The listing builds one solid part. Answer for the finished solid, in the listing's coordinates (mm). Face numbers are marked on the shaded views. A direction names the side the tool comes from. Coordinates: 2 decimals unless noted, no trailing zeros. Write each loop counter-clockwise with the first axis right and the second up, starting at its lowest first coordinate (ties: lowest second). Pieces come first, ordered by that corner, then holes.
(1) The part is cut by section C-C on y = 7.25. Determine the outline of the cut face in (x, z), plus the area to 3 significant figures.
(2) The part is cut by section B-B on y = 3.75. Determine the outline of the cut face in (x, z).
(3) Which of the six approach directions +Z, -Z, +X, -X, +Y, -Y give full straight-line access (tool end or side, diameter ignored) to the marked faces 1 and 2?
(4) Straight lines are drawn through the part: line 1 (X direction, y = 8.75, z = 1.15); line 2 (Y direction, x = -2, z = -0.9); line 3 (X direction, y = 1.5, z = 0.65). For each, find the intervals that lie inside material, in ascending order.
(5) For a pull along X with two mould halves and no side action, classify the marked faces 3, 4 and 5 as +X half, -X half, draft (parallel to the pull), parting line (faces both ways), or undercut.
(6) Given P1, Ø4, axis at x = -3, y = 2.5, coming from the -Z side, flat-ended and moving along its own axis, determine where the tip first touches the part or whether it passes through.
(7) The part is cut by section D-D on x = 5.5. Determine the outline of the cut face in (y, z).
(8) The part is cut by section A-A on z = 0.4. Determine the outline of the cut face in (x, y), plus the area to 3 significant figures.
from build123d import *

# Parameters (mm, degrees)
F1_DEPTH = 2.54
F2_R     = 2.53999
F4_D     = 4.064
F4_DEPTH = 12.5231992362
F5_D     = 4.064


# Not quite as in the source:
# - a fillet or chamfer is up to 0.001 mm smaller than in the source, because OpenCascade refuses the exact size


with BuildPart() as f1:
    # F0 (on Top) → F1 (new body, symmetric)
    with BuildSketch(Plane.XY):
        with BuildLine():
            Line((-12.5221992362, 9.4272772469), (-12.5221992362, 8.3157558613))
            Line((-12.5221992362, 8.3157558613), (-12.5221992362, 2.3621992362))
            ThreePointArc((-12.5221992362, 2.3621992362), (-11.8303270984, 0.6918721378), (-10.16, 0))
            Line((-10.16, 0), (0, 0))
            Line((0, 0), (10.16, 0))
            ThreePointArc((10.16, 0), (11.8303270984, 0.6918721378), (12.5221992362, 2.3621992362))
            Line((12.5221992362, 2.3621992362), (12.5221992362, 8.3157558613))
            Line((12.5221992362, 8.3157558613), (12.5221992362, 9.4272772469))
            Line((12.5221992362, 9.4272772469), (11.43, 9.4272772469))
            Line((11.43, 9.4272772469), (11.43, 8.3157558613))
            Line((11.43, 8.3157558613), (11.43, 2.3621992362))
            ThreePointArc((11.43, 2.3621992362), (11.0580256121, 1.464173624), (10.16, 1.0921992362))
            Line((10.16, 1.0921992362), (1.2192031136, 1.0921992362))
            Line((1.2192031136, 1.0921992362), (0, 1.0921992362))
            Line((0, 1.0921992362), (-10.16, 1.0921992362))
            ThreePointArc((-10.16, 1.0921992362), (-11.0580256121, 1.464173624), (-11.43, 2.3621992362))
            Line((-11.43, 2.3621992362), (-11.43, 8.3157558613))
            Line((-11.43, 8.3157558613), (-11.43, 9.4272772469))
            Line((-11.43, 9.4272772469), (-12.5221992362, 9.4272772469))
        make_face()
    extrude(amount=F1_DEPTH, both=True)

    # F2 (radius 2.54 in the source; OpenCascade refuses exactly that, so slightly less here)
    f2_edges = [f1.edges().sort_by_distance(p)[0] for p in [
        (-11.9761, 9.427277, 2.54),
        (-11.9761, 9.427277, -2.54),
        (11.9761, 9.427277, 2.54),
        (11.9761, 9.427277, -2.54),
    ]]
    fillet(f2_edges, radius=F2_R)

    # F4 (through all, one way)
    with BuildSketch(Plane(origin=(0, 0, 0), x_dir=(0, 1, 0), z_dir=(-1, 0, 0))):
        with Locations((6.2061757781, 0)):
            Circle(F4_D / 2)
    extrude(amount=-F4_DEPTH, mode=Mode.SUBTRACT)

    # F5 (through all)
    with Locations(Plane.YZ):
        with Locations((6.2061757781, 0)):
            Hole(F5_D / 2)


solid = f1.part
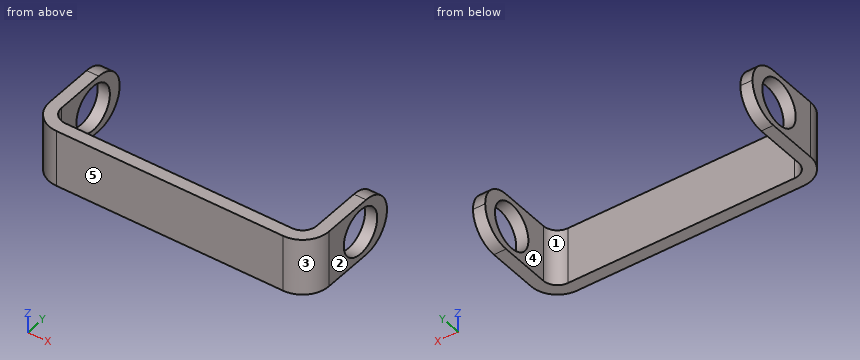
Model answer:
1. outline: (-12.52, -2.51) - (-11.43, -2.51) - (-11.43, -1.74) - (-12.52, -1.74) - close; (-12.52, 1.74) - (-11.43, 1.74) - (-11.43, 2.51) - (-12.52, 2.51) - close; (11.43, -2.51) - (12.52, -2.51) - (12.52, -1.74) - (11.43, -1.74) - close; (11.43, 1.74) - (12.52, 1.74) - (12.52, 2.51) - (11.43, 2.51) - close
1. area: 3.37 mm2
2. outline: (-12.52, -2.54) - (-11.43, -2.54) - (-11.43, 2.54) - (-12.52, 2.54) - close; (11.43, -2.54) - (12.52, -2.54) - (12.52, 2.54) - (11.43, 2.54) - close
3. face 1: +Z, -Z, +Y
3. face 2: +Z, -Z, +X, +Y, -Y
4. line 1: x = -12.52 to -11.43, 11.43 to 12.52
4. line 2: y = 0 to 1.09
4. line 3: x = -12.36 to -11.09, 11.09 to 12.36
5. face 3: +X half
5. face 4: undercut
5. face 5: draft
6. P1: stops at z = -2.54
7. outline: (0, -2.54) - (1.09, -2.54) - (1.09, 2.54) - (0, 2.54) - close
8. outline: (-12.52, 2.36) arc R2.36 ccw to (-10.16, 0) - (10.16, 0) arc R2.36 ccw to (12.52, 2.36) - (12.52, 4.21) - (11.43, 4.21) - (11.43, 2.36) arc R1.27 cw to (10.16, 1.09) - (-10.16, 1.09) arc R1.27 cw to (-11.43, 2.36) - (-11.43, 4.21) - (-12.52, 4.21) - close; (-12.52, 8.2) - (-11.43, 8.2) - (-11.43, 9.4) - (-12.52, 9.4) - close; (11.43, 8.2) - (12.52, 8.2) - (12.52, 9.4) - (11.43, 9.4) - close
8. area: 35.1 mm2
